```python
from build123d import *

# Parameters (mm, degrees)
BOSS_EXTRUDE1_DEPTH = 16
SKETCH13_R          = 11.25
CUT_EXTRUDE5_DEPTH  = 14
SKETCH14_R          = 12
CUT_EXTRUDE6_DEPTH  = 8.8
SKETCH15_R          = 9.25
CUT_EXTRUDE7_DEPTH  = 78.41184293
SKETCH17_R          = 4
CUT_EXTRUDE8_DEPTH  = 77.64224309
FILLET1_R           = 4
SKETCH18_W          = 10
SKETCH18_H          = 30
BOSS_EXTRUDE2_DEPTH = 1.2
SKETCH19_W          = 9.5
SKETCH19_H          = 36
CUT_EXTRUDE9_DEPTH  = 8.8
FILLET2_R           = 4
FILLET3_R           = 10


with BuildPart() as part:
    # Sketch2 → Boss-Extrude1 (new body)
    with BuildSketch(Plane(origin=(0, 0, 0), x_dir=(1, 0, 0), z_dir=(0, 1, 0))):
        with BuildLine():
            Line((26.74332389, 26.951705922), (22, 26.951705922))
            ThreePointArc((22, 26.951705922), (16.633883839, 25.902739872), (12.057785035, 22.91027397))
            Line((12.057785035, 22.91027397), (-5.581594366, 5.731125922))
            ThreePointArc((-5.581594366, 5.731125922), (-6.92820323, -4), (2.172503457, -7.699365476))
            Line((2.172503457, -7.699365476), (25.869771783, -1.012788831))
            ThreePointArc((25.869771783, -1.012788831), (33.364381258, 4.104419222), (36.249998435, 12.708383596))
            Line((36.249998435, 12.708383596), (36.24332389, 26.951705922))
            Line((36.24332389, 26.951705922), (36.24332389, 66.951705922))
            Line((36.24332389, 66.951705922), (26.74332389, 66.951705922))
            Line((26.74332389, 66.951705922), (26.74332389, 26.951705922))
        make_face()
    extrude(amount=BOSS_EXTRUDE1_DEPTH)

    # Sketch13 → Cut-Extrude5 (cut)
    with BuildSketch(Plane.XZ):
        with Locations(Location((22, -12.701705922, 0), (0, 0, 270))):
            Circle(SKETCH13_R)
    extrude(amount=-CUT_EXTRUDE5_DEPTH, mode=Mode.SUBTRACT)

    # Sketch14 → Cut-Extrude6 (cut)
    with BuildSketch(Plane.XZ):
        Circle(SKETCH14_R)
    extrude(amount=-CUT_EXTRUDE6_DEPTH, mode=Mode.SUBTRACT)

    # Sketch15 → Cut-Extrude7 (cut, through all)
    with BuildSketch(Plane.XZ.offset(-14)):
        with Locations(Location((22, -12.701705922, 0), (0, 0, 270))):
            Circle(SKETCH15_R)
    extrude(amount=-CUT_EXTRUDE7_DEPTH, mode=Mode.SUBTRACT)

    # Sketch17 → Cut-Extrude8 (cut, through all)
    with BuildSketch(Plane.XZ.offset(-8.8)):
        with Locations(Location((0, 0, 0), (0, 0, 270))):
            Circle(SKETCH17_R)
    extrude(amount=-CUT_EXTRUDE8_DEPTH, mode=Mode.SUBTRACT)

    # Fillet1
    fillet1_edges = [part.edges().sort_by_distance(p)[0] for p in [
        (26.74332389, 8, -26.951705922),
    ]]
    fillet(fillet1_edges, radius=FILLET1_R)

    # Sketch18 → Boss-Extrude2 (add)
    with BuildSketch(Plane(origin=(0, 16, 0), x_dir=(1, 0, 0), z_dir=(0, 1, 0))):
        with Locations((21.74332389, 51.951705922)):
            Rectangle(SKETCH18_W, SKETCH18_H)
    extrude(amount=-BOSS_EXTRUDE2_DEPTH)

    # Sketch19 → Cut-Extrude9 (cut)
    with BuildSketch(Plane.XZ):
        with Locations((31.49332389, -48.951705922)):
            Rectangle(SKETCH19_W, SKETCH19_H)
    extrude(amount=-CUT_EXTRUDE9_DEPTH, mode=Mode.SUBTRACT)

    # Fillet2
    fillet2_edges = [part.edges().sort_by_distance(p)[0] for p in [
        (31.49332389, 0, -30.951705922),
        (31.49332389, 8.8, -30.951705922),
    ]]
    fillet(fillet2_edges, radius=FILLET2_R - 0.0001)  # a hair under: the kernel refuses the full size

    # Fillet3
    fillet3_edges = [part.edges().sort_by_distance(p)[0] for p in [
        (36.24332389, 12.4, -66.951705922),
    ]]
    fillet(fillet3_edges, radius=FILLET3_R)


solid = part.part
```
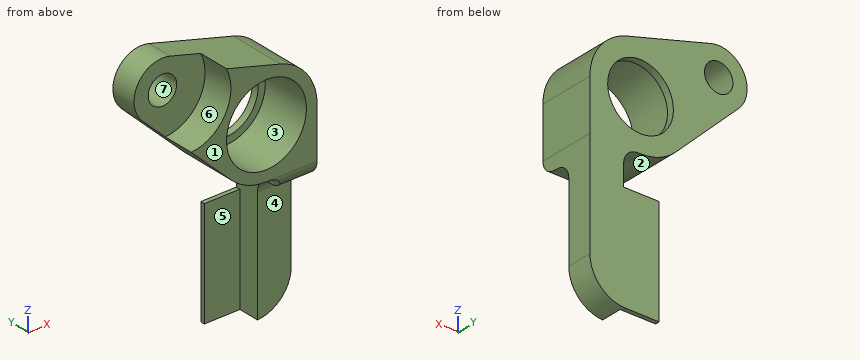
Input: part model. Units: mm. Frame: model coordinates. Face numbers are marked on the shaded views. A direction names the side the tool comes from. Give positions to 0.01 mm unless a question says otherwise; leave off trailing zeros. Write each loop counter-clockwise with the first axis right and the second up, starting at its lowest first coordinate (ties: lowest second). Pieces come first, ordered by that corner, then holes. Notation, with made-up numbers: (-33, 31) - (-29, 31) arc R10 ccw to (-29, 42) - close; hole circle Ø3 at (-15.75, 74.5). An arc over 180 degrees is marked (long way). Write item = value, one per line. Start each with the question number.
1) Reachability of the marked faces 4, 5, 6 and 7 from +Z, -Z, +X, -X, +Y, -Y: full face, straight path, thin tool, end or side. Return the list, or none.
2) Cut plane D-D (z = -39). Return loops of the section in (x, y), and give its area (3 significant figures).
3) Cut plane A-A (x = 0). Return loops of the section in (y, z), and give its area (3 significant figures).
4) Pin query (flat end, axial travel): pin 1 (8 mm diameter, centred on y = 8, z = -42, fed in from +X); pin 2 (8 mm diameter, centred on x = 7, y = 5, fed in from +Z); pin 3 (9 mm diameter, centred on y = 8, z = -41, fed in from -X). Return the tip coordinate at first contact, or that it passes through.
5) Cut plane B-B (z = -8). Return loops of the section in (x, y).
6) Draft query along X for the marked faces 1, 2 and 3. Return one class per face: pulls with the +X half, pulls with the -X half, needs draft (parallel to the pull), parting line crosses it, or undercut.
7) Material intervals for L1, parallel to X at y = 3.5, z = -7.5; L2, parallel to Z at x = 15, y = 8; L3, parallel to Z at x = 24.5, y = 8.5, sorted ascending. Write a range as [from, to].
8) Cut plane C-C (y = 1.5). Return loops of the section in (x, z), and give its area (3 significant figures).
Answers follow:
q1.face_4 = -Z, +X, -X, -Y
q1.face_5 = -Z, -X, -Y
q1.face_6 = -X, -Y
q1.face_7 = +Y, -Y
q2.outline = (16.74, 14.8) - (26.74, 14.8) - (26.74, 8.8) - (36.24, 8.8) - (36.24, 16) - (16.74, 16) - close
q2.area = 80.4 mm^2
q3.outline = (8.8, -11.17) - (16, -11.17) - (16, -4) - (8.8, -4) - close; (8.8, 4) - (16, 4) - (16, 8) - (8.8, 8) - close
q3.area = 80.4 mm^2
q4.pin_1 = 36.24
q4.pin_2 = 6.69
q4.pin_3 = 26.74
q5.outline = (-3.25, 8.8) - (8.94, 8.8) - (8.94, 0) - (11.78, 0) - (11.78, 14) - (14.03, 14) - (14.03, 16) - (-3.25, 16) - close; (29.97, 14) - (32.22, 14) - (32.22, 0) - (35.45, 0) - (35.45, 16) - (29.97, 16) - close
q6.face_1 = needs draft
q6.face_2 = pulls with the -X half
q6.face_3 = undercut
q7.L1 = [9.37, 12.02], [31.98, 35.27]
q7.L2 = [-25.11, -21.51], [-3.89, 4.08]
q7.L3 = [-27.36, -23.67], [-1.73, 1.4]
q8.outline = (0.83, -11.97) - (12.06, -22.91) arc R14.25 ccw to (22, -26.95) - (22.74, -26.95) arc R4 cw to (26.65, -30.07) - (36.24, -30.07) - (36.24, -26.95) - (36.25, -12.71) arc R14.25 ccw to (25.87, 1.01) - (10.78, 5.27) arc R12 cw to start; hole circle Ø22.5 at (22, -12.7)
q8.area = 384 mm^2
